from build123d import *

# Parameters (mm, degrees)
BASE_FLANGE1_DEPTH = 100
CUT_EXTRUDE1_REACH = 104.47
SKETCH3_R          = 2.5
FILLET1_R          = 10


# Sheet-metal steps are written as plain solids
with BuildPart() as part:
    # Sketch2 → Base-Flange1 (new body)
    with BuildSketch(Plane(origin=(0, 0, 0), x_dir=(1, 0, 0), z_dir=(0, 1, 0))):
        with BuildLine():
            Line((-10, -10), (-10, 7.75))
            ThreePointArc((-10, 7.75), (-9.340990258, 9.340990258), (-7.75, 10))
            Line((-7.75, 10), (7.75, 10))
            ThreePointArc((7.75, 10), (9.340990258, 9.340990258), (10, 7.75))
            Line((10, 7.75), (10, -10))
            Line((10, -10), (8.75, -10))
            Line((8.75, -10), (8.75, 7.75))
            ThreePointArc((8.75, 7.75), (8.457106781, 8.457106781), (7.75, 8.75))
            Line((7.75, 8.75), (-7.75, 8.75))
            ThreePointArc((-7.75, 8.75), (-8.457106781, 8.457106781), (-8.75, 7.75))
            Line((-8.75, 7.75), (-8.75, -10))
            Line((-8.75, -10), (-10, -10))
        make_face()
    extrude(amount=BASE_FLANGE1_DEPTH)

    # Cut-Extrude1: up to this face of the body (flat: up to its plane)
    cut_extrude1_end = Plane(part.part.faces().sort_by_distance((10, 50, 1.125))[0])
    # Sketch3 → Cut-Extrude1 (cut, up to the picked face)
    with BuildSketch(Plane.ZY.offset(10), mode=Mode.PRIVATE) as cut_extrude1_sk1:
        with Locations((0, 7.5)):
            Circle(SKETCH3_R)
    cut_extrude1_tool1 = split(extrude(cut_extrude1_sk1.sketch, amount=-CUT_EXTRUDE1_REACH, mode=Mode.PRIVATE), bisect_by=cut_extrude1_end, keep=Keep.BOTH, mode=Mode.PRIVATE)
    # Sketch3 → Cut-Extrude1 (cut, up to the picked face)
    with BuildSketch(Plane.ZY.offset(10), mode=Mode.PRIVATE) as cut_extrude1_sk2:
        with Locations((0, 92.5)):
            Circle(SKETCH3_R)
    cut_extrude1_tool2 = split(extrude(cut_extrude1_sk2.sketch, amount=-CUT_EXTRUDE1_REACH, mode=Mode.PRIVATE), bisect_by=cut_extrude1_end, keep=Keep.BOTH, mode=Mode.PRIVATE)
    add(cut_extrude1_tool1.solids().sort_by(Axis((-10, 7.5, 0), (1, 0, 0)))[0], mode=Mode.SUBTRACT)
    add(cut_extrude1_tool2.solids().sort_by(Axis((-10, 92.5, 0), (1, 0, 0)))[0], mode=Mode.SUBTRACT)

    # Fillet1
    fillet1_edges = [part.edges().sort_by_distance(p)[0] for p in [
        (-9.375, 0, 10),
        (9.375, 0, 10),
        (-9.375, 100, 10),
        (9.375, 100, 10),
    ]]
    fillet(fillet1_edges, radius=FILLET1_R)


solid = part.part
The listing builds one solid part. Answer for the finished solid, in the listing's coordinates (mm). A direction names the side the tool comes from. Give positions to 0.01 mm unless a question says otherwise; leave off trailing zeros. Loops run counter-clockwise (first coordinate to the right, second up) from the corner with the lowest first, then second, coordinate; pieces in that order, holes last.
Item 1: Each of these flat-tipped pins is pushed along its axis until it touches: pin 1 Ø6.5 at (y, z) = (92.5, 0) entering from +X; pin 2 Ø8 at (x, y) = (3.5, 49) entering from +Z; pin 3 Ø2 at (x, y) = (-7.5, 10.5) entering from +Z. Where does it stop, or does it pass through?
Derived:
pin 1: stops at x = 10
pin 2: stops at z = -8.75
pin 3: stops at z = -8.41
Item 2: Determine the mould class of faces 1 (the cylindrical face through (9.37, 5.06, -0.54)), 2 (the cylindrical face through (-9, 95, 0)), 3 (the flat face through (-10, 49, 1)), 4 (the cylindrical face through (-9.38, 96.99, 7.15)) for opening direction Y: +Y half, -Y half, draft (parallel to the pull), parting line (faces both ways), or undercut.
Derived:
face 1: undercut
face 2: undercut
face 3: draft
face 4: +Y half
Item 3: A cutting plane is placed at C-C (x = 4.25). Give the vertices of the cut face in (y, z), then the cut area to 3 significant figures.
Derived:
outline: (0, -10) - (100, -10) - (100, -8.75) - (0, -8.75) - close
area: 125 mm2
Item 4: A tool of negligible diameter and unlimited length cuts with its end or side. For faces 5 (the cylindrical face through (-9.38, 5.06, -0.54)), 6 (the flat face through (-8.75, 49, 1)), from which of +Z, -Z, +X, -X, +Y, -Y can it reach the whole face along a straight path? Write none if from no direction.
Derived:
face 5: +X, -X
face 6: +Z, +Y, -Y
Item 5: Find the intervals of material crossed by line 1 along X through (y, z) = (50.5, -5.5); line 2 along Z through (x, y) = (1.25, 90); line 3 along Y through (x, z) = (9, 5.5), in increasing order.
Derived:
line 1: x = -10 to -8.75, 8.75 to 10
line 2: z = -10 to -8.75
line 3: y = 1.65 to 98.35
Item 6: A cutting plane is placed at B-B (z = 8.5). Give the vertices of the cut face in (x, y), then the cut area to 3 significant figures.
Derived:
outline: (-10, 4.73) - (-8.75, 4.73) - (-8.75, 95.27) - (-10, 95.27) - close; (8.75, 4.73) - (10, 4.73) - (10, 95.27) - (8.75, 95.27) - close
area: 226 mm2
Item 7: A cutting plane is placed at D-D (z = 1.5). Give the vertices of the cut face in (x, y), then the cut area to 3 significant figures.
Derived:
outline: (-10, 0.11) - (-8.75, 0.11) - (-8.75, 5.5) - (-10, 5.5) - close; (-10, 9.5) - (-8.75, 9.5) - (-8.75, 90.5) - (-10, 90.5) - close; (-10, 94.5) - (-8.75, 94.5) - (-8.75, 99.89) - (-10, 99.89) - close; (8.75, 0.11) - (10, 0.11) - (10, 5.5) - (8.75, 5.5) - close; (8.75, 9.5) - (10, 9.5) - (10, 90.5) - (8.75, 90.5) - close; (8.75, 94.5) - (10, 94.5) - (10, 99.89) - (8.75, 99.89) - close
area: 229 mm2
Item 8: A cutting plane is placed at A-A (y = 92.5). Give the vertices of the cut face in (x, z), then the cut area to 3 significant figures.
Derived:
outline: (-10, -7.75) arc R2.25 ccw to (-7.75, -10) - (7.75, -10) arc R2.25 ccw to (10, -7.75) - (10, -2.5) - (8.75, -2.5) - (8.75, -7.75) arc R1 cw to (7.75, -8.75) - (-7.75, -8.75) arc R1 cw to (-8.75, -7.75) - (-8.75, -2.5) - (-10, -2.5) - close; (-10, 2.5) - (-8.75, 2.5) - (-8.75, 9.68) - (-10, 9.68) - close; (8.75, 2.5) - (10, 2.5) - (10, 9.68) - (8.75, 9.68) - close
area: 56.8 mm2
